Solid Edge part; units mm, degrees
sketch "Sketch1" plane through (0, 0, 0) normal (0, -1, 0) x (1, 0, 0)
  line L0 (0, 25) -> (7.0711, 17.9289)
  line L1 (14.1421, 25) -> (7.0711, 17.9289)
  line L2 (4.1421, 35) -> (14.1421, 25)
  line L3 (4.1421, 35) -> (-100, 35)
  line L4 (-100, 35) -> (-100, 25)
  line L5 (-100, 25) -> (-35, 25)
  line L6 (-35, 25) -> (-35, 0)
  line L7 (-35, 0) -> (-25, 0)
  line L8 (-25, 0) -> (-25, 25)
  line L9 (-25, 25) -> (0, 25)
extrude "Protrusion1" add sketch "Sketch1" along normal mid plane 10
fillet "Round_1" radius 5 4 edges at (3.5355, -5, 21.4645) (3.5355, 5, 21.4645) (9.1421, 5, 30) (9.1421, -5, 30)
sketch "Sketch2" plane through (-61.4645, -5, 24) normal (0, -1, 0) x (1, 0, 0)
  circle A0 centre (31.4645, -19) radius 2.25
extrude "ExtrudedCutout_1" cut sketch "Sketch2" along normal mid plane 69.4908
fillet "Round_2" radius 5 4 edges at (-25, 0, 0) (-35, 0, 0) (-25, 0, 25) (-35, 0, 25)
sketch "Sketch3" plane through (-100, 0, 43) normal (-1, 0, 0) x (0, 0, -1)
  line L0 (18, -2.5) -> (13, -2.5)
  line L1 (13, -2.5) -> (13, 2.5)
  line L2 (13, 2.5) -> (18, 2.5)
  line L3 (18, 2.5) -> (18, -2.5)
extrude "ExtrudedCutout_2" cut sketch "Sketch3" against normal blind 8
sketch "Sketch4" plane through (0, 0, 0) normal (0, -1, 0) x (1, 0, 0)
  circle A0 centre (-86, 30) radius 1.35
extrude "ExtrudedCutout_3" cut sketch "Sketch4" along normal mid plane 29.2691
fillet "Round_3" radius 2 1 edges at (-100, 2.5, 27.5)
properties material "PVC"
The listing builds one solid part. Answer for the finished solid, in the listing's coordinates (mm). A direction names the side the tool comes from. Round coordinates to 2 decimals unless told otherwise and drop trailing zeros. Order: outer loops, then holes, each group sorted by start corner. A loop starts at its lowest first (then second) coordinate and runs counter-clockwise, first axis right, second up. Notation, with made-up numbers: (81, -36.5) -> (137, -36.5) arc R34 cw to (137, 1.5) -> close; hole circle Ø4 at (-30.75, 35). An arc over 180 degrees is marked (long way). Answer as CSV lines item,"result". Start each with the question number.
(1) For a pull along Y with two mould halves and no side action, classify faces 4 (the face through (-36, 0, 23)), 5 (the face through (-96, 0, 30)), 6 (the face through (5.38, 3.5, 21.64)), 7 (the face through (5.43, -3.57, 21.69)) as +Y half, -Y half, draft (parallel to the pull), parting line (faces both ways), or undercut.
(2) Find the intervals of material crossed by probe 1 along Z at (x, y) = (-30, 0.25); probe 2 along Z at (x, y) = (-86, 1.5); probe 3 along X at (y, z) = (-2.75, 13.5), in increasing order. Write a range as from..to.
(3) The part is cut by section A-A (y = -3.5). Count the separate pieces of the cut face and the enclosed holes in it, then the cut area to 3 significant figures.
(4) The part is cut by section C-C (x = -43.5). Determine the outline of the cut face in (y, z).
(5) Flat-ended cylindrical pins translate along their axes: pin 1 Ø3 at (x, y) = (-8, 1.5) entering from -Z; pin 2 Ø2 at (x, z) = (-86, 30) entering from +Y; pin 3 Ø1 at (y, z) = (2.5, 8.5) entering from -X; pin 4 Ø3 at (x, y) = (-38, 3) entering from -Z. Find the tip coordinate at first contact, or state that the pin passes through.
(6) A tool of negligible diameter and unlimited length cuts with its end or side. For faces 1 (the face through (-99.43, 3.1, 27.54)), 2 (the face through (-24, 0, 23)), 3 (the face through (-26, 0, 2)), from which of +Z, -Z, +X, -X, +Y, -Y can it reach the whole face along a straight path? Write none if from no direction.
(7) The part is cut by section B-B (z = 15). Determine the outline of the cut face in (x, y), then the cut area to 3 significant figures.
Evaluation:
1,face 4,"draft"
1,face 5,"undercut"
1,face 6,"+Y half"
1,face 7,"-Y half"
2,probe 1,"0..2.75, 7.25..35"
2,probe 2,"25..28.65, 31.35..35"
2,probe 3,"-35..-25"
3,separate pieces,"1"
3,enclosed holes,"2"
3,area,"1,340 mm²"
4,outline,"(-5, 25) -> (5, 25) -> (5, 35) -> (-5, 35) -> close"
5,pin 1,"z = 25"
5,pin 2,"through"
5,pin 3,"x = -35"
5,pin 4,"z = 23.57"
6,face 1,"-Z, -X"
6,face 2,"-Z, +Y, -Y"
6,face 3,"-Z, +X, +Y, -Y"
7,outline,"(-35, -5) -> (-25, -5) -> (-25, 5) -> (-35, 5) -> close"
7,area,"100 mm²"
